Autodesk Inventor part; units mm, degrees
ref_plane "YZ Plane" through (0, 0, 0) normal (1, 0, 0) x (0, 1, 0)
ref_plane "XZ Plane" through (0, 0, 0) normal (0, 1, 0) x (-1, 0, 0)
ref_plane "XY Plane" through (0, 0, 0) normal (0, 0, 1) x (1, 0, 0)
sketch "Sketch1" plane through (0, 0, 0) normal (0, 0, 1) x (1, 0, 0)
  line L0 (0, 0) -> (-63.5, 0)
  line L1 (-63.5, 0) -> (-63.5, 15.875)
  line L2 (-63.5, 15.875) -> (0, 15.875)
  line L3 (0, 15.875) -> (0, 0)
  line L4 (0, 6.35) -> (-63.5, 6.35)
  line L5 (-63.5, 6.35) -> (-63.5, 9.525)
  line L6 (-63.5, 9.525) -> (0, 9.525)
  line L7 (0, 9.525) -> (0, 6.35)
  line L8 (-47.625, 15.875) -> (-15.875, 15.875)
  line L9 (-15.875, 15.875) -> (-15.875, 0)
  line L10 (-15.875, 0) -> (-47.625, 0)
  line L11 (-47.625, 0) -> (-47.625, 15.875)
  circle A0 centre (-31.75, 7.9375) radius 6.35
  circle A1 centre (-31.75, 7.9375) radius 2.5797
  line L12 (-6.35, 6.35) -> (-6.35, 9.525)
  line L13 (-57.15, 6.35) -> (-57.15, 9.525)
  point P0 (-15.875, 6.35)
  point P1 (-15.875, 9.525)
  point P2 (-47.625, 9.525)
  point P3 (-47.625, 6.35)
  dimension "d12" = 15.875
  dimension "d13" = 6.35
  dimension "d14" = 3.175
  dimension "d15" = 15.875
  dimension "d16" = 15.875
  dimension "d17" = 7.9375
  dimension "d18" = 31.75
  dimension "d19" = 12.7
  dimension "d20" = 5.1594
  dimension "d33" = 6.35
  dimension "d34" = 6.35
  dimension "d35" = 50.8
  dimension "d36" = 63.5
extrude "Extrusion1" add sketch "Sketch1" along normal blind 9.525 contours L0 L9 L4 L3 | L0 L11 L4 A0 L9 | L0 L1 L4 L11 | L4 A0 L6 L9 | L6 L9 L2 L3 | L11 L6 A0 L4 | A0 L4 A1 | L4 A1 L6 A0 | L6 A0 L11 L2 L9 | A0 L6 A1 L4 | L6 L1 L2 L11 | L6 A1 A0
extrude "Extrusion2" cut sketch "Sketch1" along normal blind 6.35 contours A0 L4 A1 | L4 A1 L6 A0 | A0 L6 A1 L4 | A1 L4 | L4 A1 L6 | L6 A1 A0 | L6 A1
sketch "Sketch2" plane through (-63.5, 15.875, 0) normal (0, 1, 0) x (1, 0, 0)
  circle A0 centre (57.15, -4.7625) radius 2.5797
  circle A1 centre (6.35, -4.7625) radius 2.5797
  line L0 (63.5, 0) -> (0, 0)
  line L1 (63.5, 0) -> (63.5, -9.525)
  line L2 (0, 0) -> (0, -9.525)
  dimension "d25" = 4.7625
  dimension "d26" = 4.7625
  dimension "d27" = 6.35
  dimension "d28" = 6.35
  dimension "d29" = 5.1594
extrude "Extrusion3" cut sketch "Sketch2" against normal through all
equation "\"d16\" = d15"
equation "\"d17\" = 0.5 * d12"
equation "\"d18\" = 0.5 * d36"
equation "\"d33\" = d34"
equation "\"d34\" = d13"
equation "\"d26\" = d25"
equation "\"d27\" = d28"
properties part number "Connector"
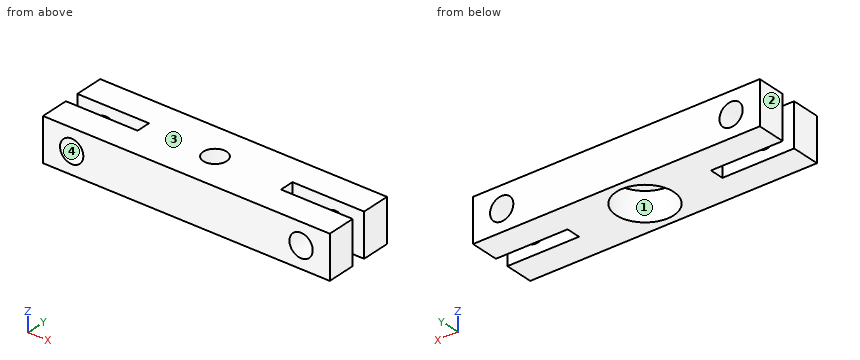
Input: part model. Units: mm. Frame: model coordinates. Face numbers are marked on the shaded views. Round coordinates to 2 decimals unless told otherwise and drop trailing zeros. Loops run counter-clockwise (first coordinate to the right, second up) from the corner with the lowest first, then second, coordinate; pieces in that order, holes last. Notation, with made-up numbers: M 70.5,35.5 L 117.5,35.5 A28 cw 117.5,62.5 Z; hole C -18,85.25 d10. An arc over 180 degrees is marked long. Answer in a Markdown table with one row per item. Add a question column.
1. Section B-B (x = -6.35). Output: boundary loops of the cut face in (y, z) (3 decimals).
2. Section C-C (x = -13). Output: boundary loops of the cut face in (y, z) (3 decimals).
3. Section A-A (z = 5.5). Give the number of separate pieces and of enclosed holes in the cut face, and give its area (3 significant figures).
4. Ray query, probe 1 along X at (y, z) = (3.25, 4.5); probe 2 along X at (y, z) = (14.5, 2.5); probe 3 along X at (y, z) = (2.75, 6). Return the intervals inside material, ascending.
5. Contact query for flat-ended pins moving along their axis: pin 1 (3 mm diameter, centred on x = -7, z = 3.5, fed in from -Y); pin 2 (4.5 mm diameter, centred on x = -57.15, z = 4.76, fed in from +Y); pin 3 (1 mm diameter, centred on y = 8, z = 5, fed in from -X) (3 decimals). Output: stop coordinate, or through.
6. Mould query, pull axis X, two halves, no side actions, for the marked faces 1, 2, 3 and 4. Classes: released by +X, released by -X, zero draft, split by the parting line, or undercut.
Values follow:
| question | item | result |
|---|---|---|
| 1 | outline | M 0,0 L 6.35,0 L 6.35,2.183 L 0,2.183 Z; M 0,7.342 L 6.35,7.342 L 6.35,9.525 L 0,9.525 Z; M 9.525,0 L 15.875,0 L 15.875,2.183 L 9.525,2.183 Z; M 9.525,7.342 L 15.875,7.342 L 15.875,9.525 L 9.525,9.525 Z |
| 2 | outline | M 0,0 L 6.35,0 L 6.35,9.525 L 0,9.525 Z; M 9.525,0 L 15.875,0 L 15.875,9.525 L 9.525,9.525 Z |
| 3 | separate pieces | 5 |
| 3 | enclosed holes | 1 |
| 3 | area | 655 mm^2 |
| 4 | probe 1 | -63.5 to -59.72, -54.58 to -36.03, -27.47 to -8.92, -3.78 to 0 |
| 4 | probe 2 | -63.5 to -58.39, -55.91 to -7.59, -5.11 to 0 |
| 4 | probe 3 | -63.5 to -59.41, -54.89 to -35.41, -28.09 to -8.61, -4.09 to 0 |
| 5 | pin 1 | y = 0 |
| 5 | pin 2 | through |
| 5 | pin 3 | x = -47.625 |
| 6 | face 1 | undercut |
| 6 | face 2 | released by -X |
| 6 | face 3 | zero draft |
| 6 | face 4 | undercut |
